Here's how the part is built. I have some questions about the finished solid (model axes, mm). Face numbers are marked on the shaded views. Coordinates: 2 decimals unless noted, no trailing zeros. Write each loop counter-clockwise with the first axis right and the second up, starting at its lowest first coordinate (ties: lowest second). Pieces come first, ordered by that corner, then holes.
Item 1: I want a section at A-A (y = 0). Please give me the cut outline in (x, z).
Item 2: I want a section at B-B (x = 0). Please give me the cut outline in (y, z), and give its area (3 significant figures).
Item 3: If we mould it in two halves opening along X, with no side actions, what happens to the marked faces 1 and 2? For each: pulls with the +X half, pulls with the -X half, needs draft (parallel to the pull), parting line crosses it, or undercut.
Item 4: I'm going to push flat-ended pins straight in: P1, Ø3, axis at x = -7, z = 127.5, coming from the -Y side; P2, Ø5, axis at x = 0, z = 145, coming from the -Y side. Where does each tip first touch, or does it pass through?
Item 5: Please list where these lines run through material, in increasing order: line 1 (Z direction, x = 0, y = 9); line 2 (Y direction, x = -0.5, z = 68); line 3 (X direction, y = 7.75, z = 104).
Item 6: I want a section at D-D (z = 109.5). Please give me the cut outline in (x, y), and give its area (3 significant figures).
Item 7: I want a section at C-C (z = 145). Please give me the cut outline in (x, y), and give its area (3 significant figures).
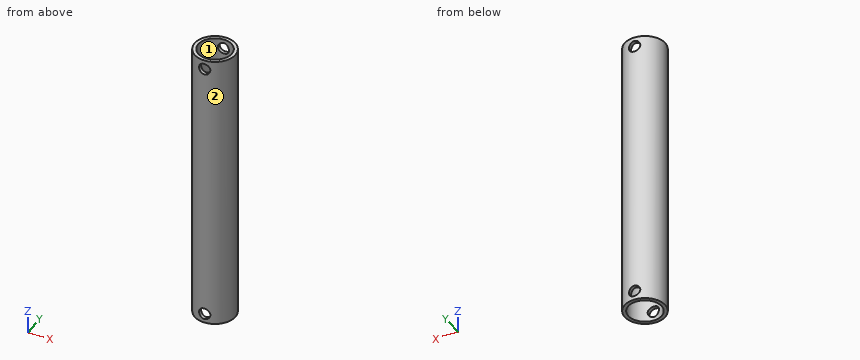
Autodesk Inventor part; units mm, degrees
ref_plane "Work Plane1" through (0, -10.75, 0) normal (0, 1, 0) x (-1, 0, 0)
ref_plane "YZ Plane" through (0, 0, 0) normal (1, 0, 0) x (0, 1, 0)
ref_plane "XY Plane" through (0, 0, 0) normal (0, 0, 1) x (1, 0, 0)
sketch "Sketch1" plane through (0, 0, 0) normal (0, 0, 1) x (1, 0, 0)
  circle A0 centre (0, 0) radius 10.75
  circle A1 centre (0, 0) radius 8.85
  dimension "d0" = 21.5
  dimension "d1" = 17.7
extrude "Extrusion1" add sketch "Sketch1" along normal blind 150
ref_plane "Work Plane1" through (0, -10.75, 0) normal (0, 1, 0) x (-1, 0, 0)
sketch "Sketch2" plane through (0, -10.75, 0) normal (0, 1, 0) x (-1, 0, 0)
  circle A0 centre (0, 5) radius 3
  line L0 (0, -39.6) -> (0, 237.6)
  line L1 (10.75, 0) -> (-10.75, 0)
  circle A1 centre (0, 145) radius 3
  line L2 (10.75, 150) -> (-10.75, 150)
  point P0 (0, 0)
  dimension "d4" = 6
  dimension "d5" = 5
  dimension "d8" = 6
  dimension "d9" = 5
extrude "Extrusion2" cut sketch "Sketch2" along normal through all
properties part number "Shifter Post" material "PVC-Piping"
Answer:
1. outline: (-10.75, 0) - (-8.85, 0) - (-8.85, 150) - (-10.75, 150) - close; (8.85, 0) - (10.75, 0) - (10.75, 150) - (8.85, 150) - close
2. outline: (-10.75, 0) - (-8.85, 0) - (-8.85, 2) - (-10.75, 2) - close; (-10.75, 8) - (-8.85, 8) - (-8.85, 142) - (-10.75, 142) - close; (-10.75, 148) - (-8.85, 148) - (-8.85, 150) - (-10.75, 150) - close; (8.85, 0) - (10.75, 0) - (10.75, 2) - (8.85, 2) - close; (8.85, 8) - (10.75, 8) - (10.75, 142) - (8.85, 142) - close; (8.85, 148) - (10.75, 148) - (10.75, 150) - (8.85, 150) - close
2. area: 524 mm2
3. face 1: undercut
3. face 2: parting line crosses it
4. P1: stops at y = -9.24
4. P2: passes through
5. line 1: z = 0 to 2, 8 to 142, 148 to 150
5. line 2: y = -10.74 to -8.84, 8.84 to 10.74
5. line 3: x = -7.45 to -4.27, 4.27 to 7.45
6. outline: circle Ø21.5 at (0, 0); hole circle Ø17.7 at (0, 0)
6. area: 117 mm2
7. outline: (-3, -10.32) - (-3, -8.33) arc R8.85 cw to (-3, 8.33) - (-3, 10.32) arc R10.75 ccw to start; (3, -10.32) arc R10.75 ccw to (3, 10.32) - (3, 8.33) arc R8.85 cw to (3, -8.33) - close
7. area: 93.8 mm2
